Part print with two shaded views. Sizes in mm from the minimum x, y, z corner. Round coordinates to 2 decimals unless told otherwise and drop trailing zeros. Write each loop counter-clockwise with the first axis right and the second up, starting at its lowest first coordinate (ties: lowest second). Pieces come first, ordered by that corner, then holes. Notation, with made-up numbers: (-12.5, 12) - (14.5, 12) arc R21 ccw to (14.5, 51) - close; hole circle Ø11 at (-3, 54.25). An arc over 180 degrees is marked (long way). Answer as a JSON object with one key per item and string values. Group by question number.
Item 1: Slice it at B-B, the plane x = 34. List the corners of the cut face in (y, z), then the cut area to 3 significant figures.
Item 2: Slice it at A-A, the plane z = 3. List the corners of the cut face in (x, y).
Item 3: Slice it at C-C, the plane y = 10. List the corners of the cut face in (x, z), then the cut area to 3 significant figures.
Item 4: Probe line 1 (Y direction, x = 34.5, z = 16.5); line 2 (Y direction, x = 27, z = 19.5); line 3 (X direction, y = 12.5, z = 3.75). List the from-to ranges inside material, lowest first. Write a range as from..to.
Item 5: Flat gauge pins, fed straight in: pin 1 (1.5 mm diameter, centred on x = 4, z = 11.5, fed in from +Y); pin 2 (10 mm diameter, centred on x = 33.5, z = 6, fed in from +Y); pin 3 (3 mm diameter, centred on y = 11, z = 4, fed in from +X). Where does each tip first touch, or does it go through?
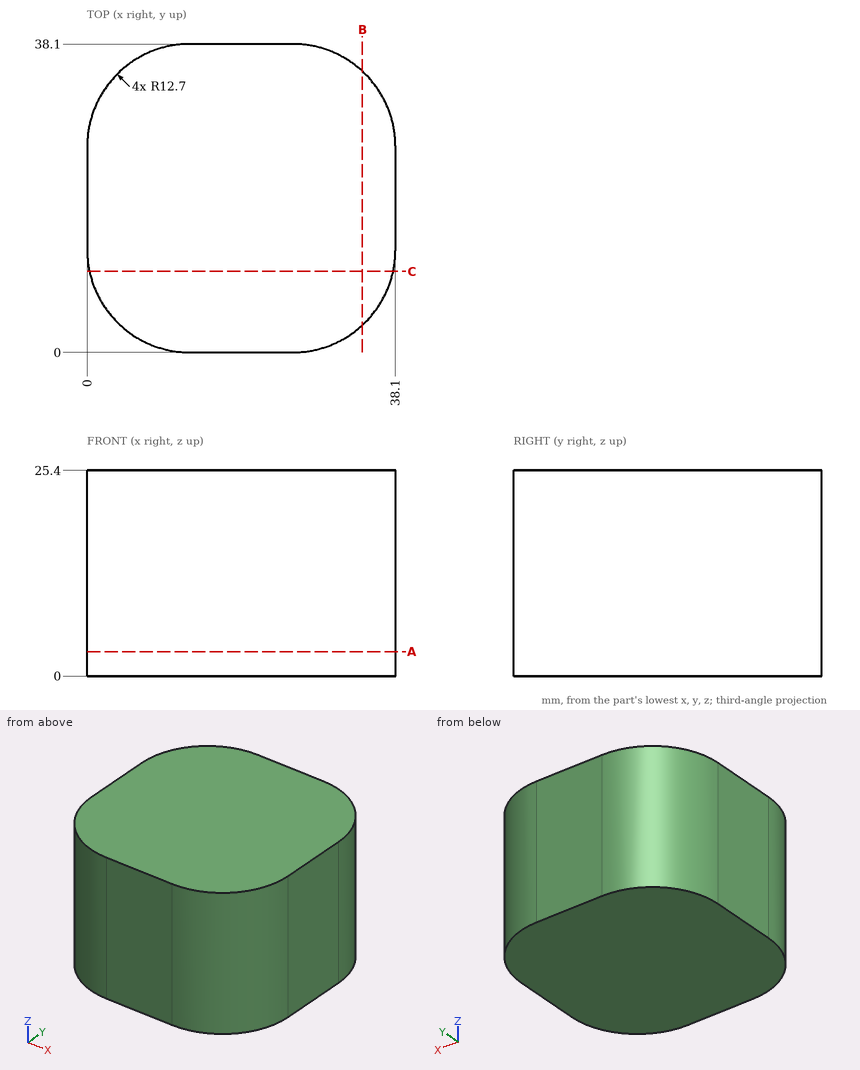
Geometry says:
{
 "1": {"outline": "(3.35, 0) - (34.75, 0) - (34.75, 25.4) - (3.35, 25.4) - close", "area": "797 mm^2"},
 "2": {"outline": "(0, 12.7) arc R12.7 ccw to (12.7, 0) - (25.4, 0) arc R12.7 ccw to (38.1, 12.7) - (38.1, 25.4) arc R12.7 ccw to (25.4, 38.1) - (12.7, 38.1) arc R12.7 ccw to (0, 25.4) - close"},
 "3": {"outline": "(0.29, 0) - (37.81, 0) - (37.81, 25.4) - (0.29, 25.4) - close", "area": "953 mm^2"},
 "4": {"line 1": "y = 3.84..34.26", "line 2": "y = 0.1..38", "line 3": "x = 0..38.1"},
 "5": {"pin 1": "stops at y = 35.3", "pin 2": "stops at y = 37.72", "pin 3": "stops at x = 38.1"}
}
